Autodesk Inventor part; units mm, degrees
sketch "Skizze1" plane through (0, 0, 0) normal (0, 0, 1) x (1, 0, 0)
  line L0 (-5, 5) -> (5, 5)
  line L1 (5, 5) -> (5, -5)
  line L2 (5, -5) -> (-5, -5)
  line L3 (-5, -5) -> (-5, 5)
  line L4 (-7, 0) -> (7, 0)
  line L5 (0, 7) -> (0, -7)
  point P0 (0, 0)
  dimension "d0" = 10
  dimension "d1" = 10
extrude "Extrusion1" add sketch "Skizze1" along normal mid plane 3
sketch "Skizze2" plane through (0, 0, 1.5) normal (0, 0, 1) x (1, 0, 0)
  circle A0 centre (0, 0) radius 1.5
  dimension "d4" = 3
extrude "Extrusion2" cut sketch "Skizze2" against normal blind 3
thread "Gewinde1"
chamfer "Fase1" distance 2 angle 45 4 edges at (5, 5, 0) (-5, 5, 0) (5, -5, 0) (-5, -5, 0)
properties part number "RadAxeVorneSicherung"
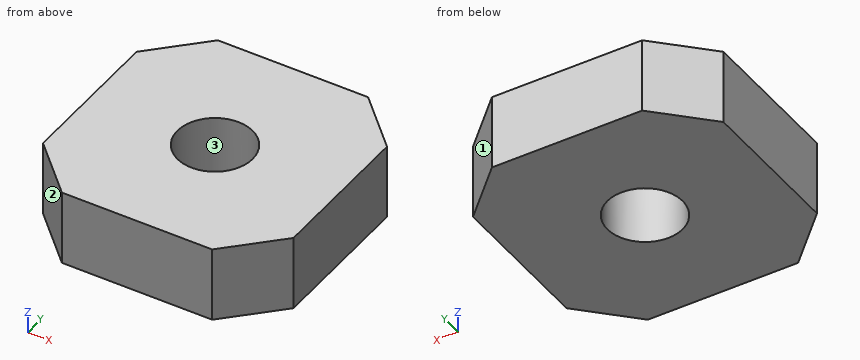
Design review of the part built by this model. Coordinates are the model's own, in mm. Face numbers are marked on the shaded views. Give positions to 0.01 mm unless a question says otherwise; leave off trailing zeros. Write each loop counter-clockwise with the first axis right and the second up, starting at its lowest first coordinate (ties: lowest second). Pieces come first, ordered by that corner, then holes. Notation, with made-up numbers: M -32,41.5 L 11,41.5 A24 ccw 11,54.5 Z; hole C -5.75,31 d9. An arc over 180 degrees is marked long. Return JSON: item names as keys, results as strings. Group by question number.
Item 1: Take a section at A-A (y = 0). Give the boundary of the cut face in (x, z), plus the area to 3 significant figures.
Item 2: Take a section at B-B (z = 0.4). Give the boundary of the cut face in (x, y), plus the area to 3 significant figures.
Item 3: The part is to be moulded in two halves that separate along Y. For the marked faces 1, 2 and 3, say which applies: pulls with the +Y half, pulls with the -Y half, needs draft (parallel to the pull), parting line crosses it, or undercut.
Item 4: Wall thickness on line 1 along Y through (x, z) = (0, -0.6); line 2 along X through (y, z) = (-0.5, 1); line 3 along Y through (x, z) = (1.25, -0.3): over which ranges is each line inside the solid? List them lowest first.
Item 5: Take a section at D-D (y = 3.25). Give the boundary of the cut face in (x, z), plus the area to 3 significant figures.
Return value:
{
 "1": {"outline": "M -5,-1.5 L -1.5,-1.5 L -1.5,1.5 L -5,1.5 Z; M 1.5,-1.5 L 5,-1.5 L 5,1.5 L 1.5,1.5 Z", "area": "21.0 mm2"},
 "2": {"outline": "M -5,-3 L -3,-5 L 3,-5 L 5,-3 L 5,3 L 3,5 L -3,5 L -5,3 Z; hole C 0,0 d3", "area": "84.9 mm2"},
 "3": {"face 1": "pulls with the +Y half", "face 2": "pulls with the -Y half", "face 3": "undercut"},
 "4": {"line 1": "y = -5 to -1.5, 1.5 to 5", "line 2": "x = -5 to -1.41, 1.41 to 5", "line 3": "y = -5 to -0.83, 0.83 to 5"},
 "5": {"outline": "M -4.75,-1.5 L 4.75,-1.5 L 4.75,1.5 L -4.75,1.5 Z", "area": "28.5 mm2"}
}
